from build123d import *

# Parameters (mm, degrees)
ENL_V_START             = -5.5
ESQUISSE2_W             = 11.618950038
ESQUISSE2_H             = 44.4
ENL_V_MAT_EXTRU_1_DEPTH = 5.2
ENL_V_MAT_EXTRU_2_DEPTH = 10.7
ESQUISSE6_R             = 3.5
ENL_V_MAT_EXTRU_3_DEPTH = 120
CHANFREIN1_SIZE         = 1


with BuildPart() as part:
    # Esquisse1 → Révolution1 (revolve)
    with BuildSketch(Plane.XY):
        Polygon((0, 0), (-7, 0), (-8, 1), (-8, 50), (-7.75, 50), (-7.75, 51.3), (-8.4, 51.3), (-8.4, 57.3), (-8.6, 57.3), (-8.6, 66.3), (-8.33, 66.3), (-8.33, 68.3), (-9.7, 68.3), (-9.7, 80.3), (-8.15, 80.3), (-8.15, 96.5), (-7.5, 96.5), (-7.5, 97.5), (-8.15, 97.5), (-8.15, 99), (-7.5, 99), (-7.5, 106), (-6.5, 107), (0, 107), align=None)
    revolve(axis=Axis((0, 107, 0), (0, -1, 0)))

    # Esquisse2 → Enlèv. mat.-Extru.1 (cut, through all)
    with BuildSketch(Plane.XY.offset(ENL_V_START)):
        with Locations((0, 24.9)):
            Rectangle(ESQUISSE2_W, ESQUISSE2_H)
    extrude(amount=-ENL_V_MAT_EXTRU_1_DEPTH, mode=Mode.SUBTRACT)

    # Esquisse5 → Enlèv. mat.-Extru.2 (cut, through all)
    with BuildSketch(Plane(origin=(0, 0, 0), x_dir=(0, 0, -1), z_dir=(1, 0, 0))):
        with BuildLine():
            ThreePointArc((0, 76.3), (-3.5, 72.8), (0, 69.3))
            ThreePointArc((0, 69.3), (3.5, 72.8), (0, 76.3))
        make_face()
    extrude(amount=ENL_V_MAT_EXTRU_2_DEPTH, mode=Mode.SUBTRACT)

    # Esquisse6 → Enlèv. mat.-Extru.3 (cut)
    with BuildSketch(Plane.XZ):
        Circle(ESQUISSE6_R)
    extrude(amount=-ENL_V_MAT_EXTRU_3_DEPTH, mode=Mode.SUBTRACT)

    # Chanfrein1
    chanfrein1_edges = [part.edges().sort_by_distance(p)[0] for p in [
        (-3.5, 0, 0),
    ]]
    chamfer(chanfrein1_edges, length=CHANFREIN1_SIZE)


solid = part.part
Can you work these out from the model? Positions are in its coordinate system, mm. A direction names the side the tool comes from. Coordinates: 2 decimals unless noted, no trailing zeros. Order: outer loops, then holes, each group sorted by start corner. A loop starts at its lowest first (then second) coordinate and runs counter-clockwise, first axis right, second up. Notation, with made-up numbers: M -15.75,10.5 L 8.25,10.5 A19 cw 8.25,25.5 Z; hole C 55,72.25 d6. An arc over 180 degrees is marked long. Answer as CSV lines item,"result".
(1) I'm going to push flat-ended pins straight in: pin 1 (6 mm diameter, centred on x = 3.5, y = 94, fed in from +Z); pin 2 (5 mm diameter, centred on y = 26, z = 4, fed in from +X); pin 3 (6 mm diameter, centred on x = -6.5, y = 87.5, fed in from -Z). Where does each tip first touch, or does it pass through?
Geometry check:
pin 1,"z = 8.13"
pin 2,"x = 7.86"
pin 3,"z = -7.36"
(2) On a 3-axis mill with a long thin cutter (end or side, diameter ignored), from which of +Z, -Z, +X, -X, +Y, -Y can I reach the whole of each face in a straight line? I mean faces 4 (the cylindrical face through (-8.012, 54.342, -2.523)), 5 (the cylindrical face through (-9.252, 74.384, -2.914)), 6 (the flat face through (-3, 107, 3)), 7 (the cylindrical face through (7.493, 97.007, -0.33)), 8 (the flat face through (0, 47.1, -6)). Say none if no direction works.
Geometry check:
face 4,"-Y"
face 5,"+Y, -Y"
face 6,"+Z, -Z, +X, -X, +Y"
face 7,"none"
face 8,"-Z, +X, -X"
(3) Suppose I cut it at D-D on y = 72.8. Please give me the cut outline in (x, z), plus the area to 3 significant figures.
Geometry check:
outline,"M 0,-3.5 A3.5 cw 0,3.5 L 9.05,3.5 A9.7 ccw long 9.05,-3.5 Z"
area,"210 mm^2"
(4) If we mould it in two halves opening along Z, with no side actions, what happens to faces 1 (the cylindrical face through (-7.945, 67.314, -2.502)), 2 (the cylindrical face through (3.233, 53.258, -1.341)), 3 (the flat face through (5, 80.3, -7))? For each: released by +Z, released by -Z, zero draft, split by the parting line, or undercut.
Geometry check:
face 1,"split by the parting line"
face 2,"undercut"
face 3,"zero draft"
(5) Please list where these lines run through material, in increasing order: L1, parallel to Y at x = 8.5, z = -1; L2, parallel to Z at x = 0, y = 80.5; L3, parallel to Y at x = -3.5, z = 7.
Geometry check:
L1,"57.3 to 66.3, 68.3 to 69.45, 76.15 to 80.3"
L2,"-8.15 to -3.5, 3.5 to 8.15"
L3,"0.83 to 50, 51.3 to 96.5, 97.5 to 99"
(6) Suppose I cut it at A-A on y = 91. Please give me the cut outline in (x, z), plus the area to 3 significant figures.
Geometry check:
outline,"C 0,0 d16.3; hole C 0,0 d7"
area,"170 mm^2"
(7) Suppose I cut it at C-C on y = 27. Please give me the cut outline in (x, z).
Geometry check:
outline,"M -5.81,-5.5 L 5.81,-5.5 A8 ccw long Z; hole C 0,0 d7"
(8) Suppose I cut it at B-B on z = -2. Count the separate pieces of the cut face and the enclosed holes in it, plus the area to 3 significant figures.
Geometry check:
separate pieces,"3"
enclosed holes,"0"
area,"1,060 mm^2"
